from build123d import *

# Parameters (mm, degrees)
F0_R     = 11
F1_DEPTH = 7


with BuildPart() as f1:
    # F0 (on Top) → F1 (new body)
    with BuildSketch(Plane.XY):
        with BuildLine():
            ThreePointArc((3.804226, 28.291796), (0, 31.055728), (-3.804226, 28.291796))
            Line((-3.804226, 28.291796), (-8.082504, 15.124612))
            ThreePointArc((-8.082504, 15.124612), (-9.535589, 13.124612), (-11.88673, 12.36068))
            Line((-11.88673, 12.36068), (-25.731527, 12.36068))
            ThreePointArc((-25.731527, 12.36068), (-29.535753, 9.596748), (-28.082668, 5.124612))
            Line((-28.082668, 5.124612), (-16.881992, -3.013156))
            ThreePointArc((-16.881992, -3.013156), (-15.428907, -5.013156), (-15.428907, -7.485292))
            Line((-15.428907, -7.485292), (-19.707184, -20.652476))
            ThreePointArc((-19.707184, -20.652476), (-18.254099, -25.124612), (-13.551817, -25.124612))
            Line((-13.551817, -25.124612), (-2.351141, -16.986844))
            ThreePointArc((-2.351141, -16.986844), (0, -16.222912), (2.351141, -16.986844))
            Line((2.351141, -16.986844), (13.551817, -25.124612))
            ThreePointArc((13.551817, -25.124612), (18.254099, -25.124612), (19.707184, -20.652476))
            Line((19.707184, -20.652476), (15.428907, -7.485292))
            ThreePointArc((15.428907, -7.485292), (15.428907, -5.013156), (16.881992, -3.013156))
            Line((16.881992, -3.013156), (28.082668, 5.124612))
            ThreePointArc((28.082668, 5.124612), (29.535753, 9.596748), (25.731527, 12.36068))
            Line((25.731527, 12.36068), (11.88673, 12.36068))
            ThreePointArc((11.88673, 12.36068), (9.535589, 13.124612), (8.082504, 15.124612))
            Line((8.082504, 15.124612), (3.804226, 28.291796))
        make_face()
        Circle(F0_R, mode=Mode.SUBTRACT)
    extrude(amount=-F1_DEPTH)


solid = f1.part
Design review of the part built by this model. Coordinates are the model's own, in mm. A direction names the side the tool comes from. Round coordinates to 2 decimals unless told otherwise and drop trailing zeros. Write each loop counter-clockwise with the first axis right and the second up, starting at its lowest first coordinate (ties: lowest second). Pieces come first, ordered by that corner, then holes. Notation, with made-up numbers: M -14,-28.5 L 13,-28.5 A17 cw 13,-14.5 Z; hole C -13.75,30 d8. An arc over 180 degrees is marked long. One line per item, written item: value. Start each with the question number.
1. Take a section at A-A on z = -4. State the section outline as (x, y) points.
2. Take a section at D-D on y = 26.5. State the section outline as (x, z) points.
3. Draft analysis for pull direction X (two halves, no side actions). For faces 6 (the face through (-18.311, -25.083, -3.451)), 7 (the face through (9.564, 13.104, -3.451)), 8 (the face through (-22.56, 1.11, -3.45)), state which applies: pulls with the +X half, pulls with the -X half, needs draft (parallel to the pull), parting line crosses it, or undercut.
4. Take a section at C-C on y = 8.5. State the section outline as (x, z) points, then the cut area to 3 significant figures.
5. To check wall thickness, follow probe 1 along Y at (x, z) = (-3.5, -3.25); probe 2 along Y at (x, z) = (2.5, -5) (3 decimals); probe 3 along X at (y, z) = (6, -5.75). State the ranges of each line that lie inside material, in increasing order. Write a range as from..to.
6. Take a section at B-B on x = 0. State the section outline as (y, z) points, then the cut area to 3 significant figures.
7. Clearance check with flat-ended pins moving along their axes: P1, Ø3, axis at x = -7.5, z = -2.5, coming from the -Y side; P2, Ø3, axis at x = -13, z = -5.5, coming from the -Y side; P3, Ø3, axis at x = 12.5, z = -4, coming from the +Y side; P4, Ø4, axis at x = -11.5, y = -2.5, coming from the +Z side. State where each tip first meets the part, or that it passes through.
8. For faces 1 (the face through (-2.38, -10.74, -3.45)), 2 (the face through (7.873, -20.999, -3.451)), 3 (the face through (6, -10, -7)), 4 (the face through (22.404, 0.999, -3.451)), 5 (the face through (-17.54, -13.98, -3.45)), list the 3-axis set-ups (+Z, -Z, +X, -X, +Y, -Y) from which the entire face can be reached by the end or side of a thin tool; tool diameter is ignored.
Computed:
1. outline: M -28.08,5.12 L -16.88,-3.01 A4 cw -15.43,-7.49 L -19.71,-20.65 A4 ccw -13.55,-25.12 L -2.35,-16.99 A4 cw 2.35,-16.99 L 13.55,-25.12 A4 ccw 19.71,-20.65 L 15.43,-7.49 A4 cw 16.88,-3.01 L 28.08,5.12 A4 ccw 25.73,12.36 L 11.89,12.36 A4 cw 8.08,15.12 L 3.8,28.29 A4 ccw -3.8,28.29 L -8.08,15.12 A4 cw -11.89,12.36 L -25.73,12.36 A4 ccw Z; hole C 0,0 d22
2. outline: M -4.39,-7 L 4.39,-7 L 4.39,0 L -4.39,0 Z
3. face 6: undercut
3. face 7: pulls with the +X half
3. face 8: pulls with the -X half
4. outline: M -29.73,-7 L -6.98,-7 L -6.98,0 L -29.73,0 Z; M 6.98,-7 L 29.73,-7 L 29.73,0 L 6.98,0 Z
4. area: 318 mm²
5. probe 1: y = -17.82..-10.43, 10.43..28.99
5. probe 2: y = -17.095..-10.712, 10.712..30.178
5. probe 3: x = -28.96..-9.22, 9.22..28.96
6. outline: M -16.22,-7 L -11,-7 L -11,0 L -16.22,0 Z; M 11,-7 L 31.06,-7 L 31.06,0 L 11,0 Z
6. area: 177 mm²
7. P1: stops at y = -21.82
7. P2: stops at y = -25.63
7. P3: stops at y = 12.46
7. P4: stops at z = 0
8. face 1: +Z, -Z
8. face 2: +Z, -Z, -Y
8. face 3: -Z, +X, -X, +Y, -Y
8. face 4: +Z, -Z, +X
8. face 5: +Z, -Z, -X
